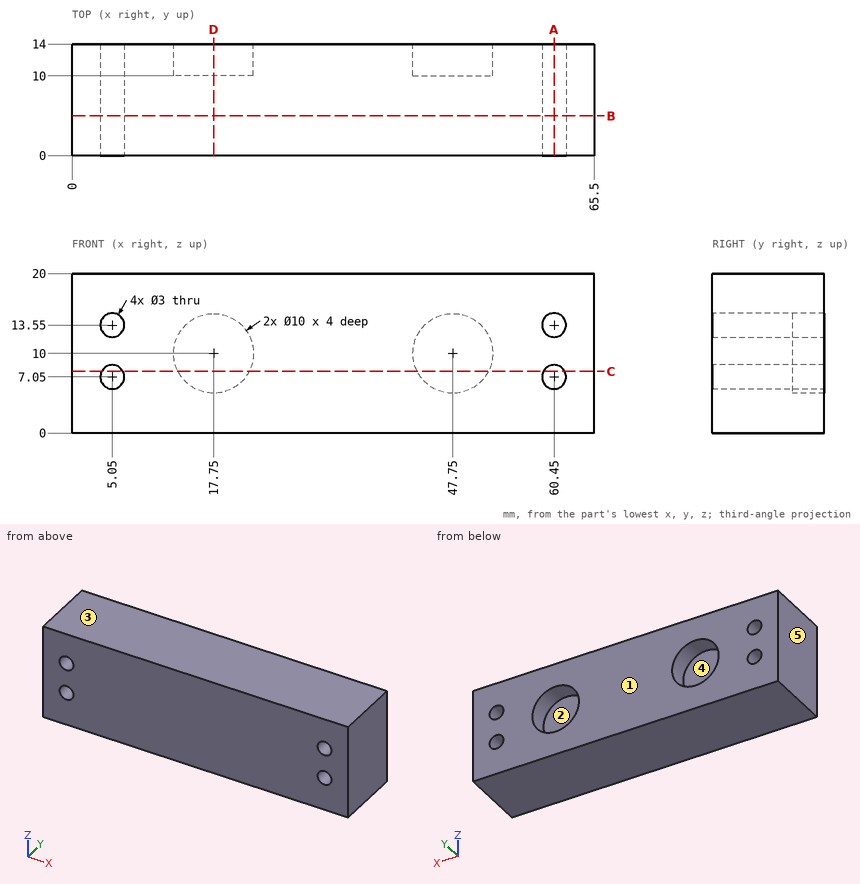
Drawing for the job (mm, zero at the part's lowest x, y, z). A direction names the side the tool comes from. Round coordinates to 2 decimals unless told otherwise and drop trailing zeros. Loops run counter-clockwise (first coordinate to the right, second up) from the corner with the lowest first, then second, coordinate; pieces in that order, holes last. Notation, with made-up numbers: (-30.5, 88.25) -> (20.5, 88.25) arc R23 cw to (20.5, 104.25) -> close; hole circle Ø4 at (-7.5, -4). An arc over 180 degrees is marked (long way). Answer in a Markdown table with one row per item.
Item 1: Saw through at A-A (x = 60.45). Write the cut outline in (y, z), and give its area (3 significant figures).
Answers below:
| item | result |
|---|---|
| outline | (0, 0) -> (14, 0) -> (14, 5.55) -> (0, 5.55) -> close; (0, 8.55) -> (14, 8.55) -> (14, 12.05) -> (0, 12.05) -> close; (0, 15.05) -> (14, 15.05) -> (14, 20) -> (0, 20) -> close |
| area | 196 mm² |
Item 2: Saw through at B-B (y = 5). Write the cut outline in (x, z), and give its area (3 significant figures).
Answers below:
| item | result |
|---|---|
| outline | (0, 0) -> (65.5, 0) -> (65.5, 20) -> (0, 20) -> close; hole circle Ø3 at (5.05, 7.05); hole circle Ø3 at (5.05, 13.55); hole circle Ø3 at (60.45, 7.05); hole circle Ø3 at (60.45, 13.55) |
| area | 1,280 mm² |
Item 3: Drill centre lines: L1, parallel to X at y = 12.95, z = 10; L2, parallel to X at y = 3.25, z = 7.05; L3, parallel to X at y = 11, z = 7.05. Where is each one in solid material? Low to high. Write a range as [from, to].
Answers below:
| item | result |
|---|---|
| L1 | x = [0, 12.75], [22.75, 42.75], [52.75, 65.5] |
| L2 | x = [0, 3.55], [6.55, 58.95], [61.95, 65.5] |
| L3 | x = [0, 3.55], [6.55, 13.71], [21.79, 43.71], [51.79, 58.95], [61.95, 65.5] |
Item 4: Pin check, flat tip, straight feed: pin 1 (2.5 mm diameter, centred on x = 5.05, z = 13.55, fed in from +Y). Stop position of the tip, or through.
Answers below:
| item | result |
|---|---|
| pin 1 | passes through |
Item 5: Mould opens along X. For the marked faces 3, 4 and 5 say: +X half, -X half, draft (parallel to the pull), parting line (faces both ways), or undercut.
Answers below:
| item | result |
|---|---|
| face 3 | draft |
| face 4 | undercut |
| face 5 | -X half |
Item 6: Saw through at C-C (z = 7.75). Write the cut outline in (x, y), and give its area (3 significant figures).
Answers below:
| item | result |
|---|---|
| outline | (0, 0) -> (3.72, 0) -> (3.72, 14) -> (0, 14) -> close; (6.38, 0) -> (59.12, 0) -> (59.12, 14) -> (52.22, 14) -> (52.22, 10) -> (43.28, 10) -> (43.28, 14) -> (22.22, 14) -> (22.22, 10) -> (13.28, 10) -> (13.28, 14) -> (6.38, 14) -> close; (61.78, 0) -> (65.5, 0) -> (65.5, 14) -> (61.78, 14) -> close |
| area | 771 mm² |
Item 7: Which spindle directions (+Z, -Z, +X, -X, +Y, -Y) get a long thin tool onto all of the face, cutting with end or side? Do the marked faces 1 and 2. Say none if no direction does.
Answers below:
| item | result |
|---|---|
| face 1 | +Z, -Z, +X, -X, +Y |
| face 2 | +Y |
Item 8: Saw through at D-D (x = 17.75). Write the cut outline in (y, z).
Answers below:
| item | result |
|---|---|
| outline | (0, 0) -> (14, 0) -> (14, 5) -> (10, 5) -> (10, 15) -> (14, 15) -> (14, 20) -> (0, 20) -> close |
